Source: CAD feature listing. Evaluate the final solid. Frame: model axes, mm. Round coordinates to 2 decimals unless told otherwise and drop trailing zeros. Order: outer loops, then holes, each group sorted by start corner. A loop starts at its lowest first (then second) coordinate and runs counter-clockwise, first axis right, second up. Notation, with made-up numbers: (-34, 69.5) - (21, 69.5) arc R13 ccw to (21, 79.5) - close; hole circle Ø7 at (48, 33.5). An arc over 180 degrees is marked (long way). Use one line per item in the form item = value. Start each with the question number.
Q1. Pin query (flat end, axial travel): pin 1 Ø5 at (y, z) = (47, -16) entering from +X; pin 2 Ø5 at (y, z) = (79, 518.5) entering from +X; pin 3 Ø22.5 at (x, y) = (0, 0) entering from -Z; pin 4 Ø6 at (x, z) = (55, 151) entering from -Y. Return the tip coordinate at first contact, or that it passes through.
Q2. Cut plane A-A, the plane z = 119.5. Return the cut outline in (x, y), and give its area (3 significant figures).
Q3. Ray query, line 1 (Y direction, x = 0, z = 490); line 2 (X direction, y = -6.5, z = 469.5); line 3 (Y direction, x = 0, z = -408.75). Return the intervals inside material, ascending. Write a range as [from, to].
Q4. Draft query along Y for faces 1 (the cylindrical face through (-32.22, 245.394, 493.34)), 2 (the conical face through (-22.371, 100.745, -254.267)), 3 (the flat face through (-242, 57, 1000)). Return one class per face: released by +Y, released by -Y, zero draft, split by the parting line, or undercut.
Q5. Cut plane B-B, the plane z = -322. Return the cut outline in (x, y), and give its area (3 significant figures).
from build123d import *

# Parameters (mm, degrees)
F0_R     = 250
F1_DEPTH = 1000
F2_R     = 250
F4_T     = -2.5
F5_R     = 12.5
F6_DEPTH = 433.0137019922


# Not quite as in the source:
# - an extrude whose draft closes it to a point is written as a loft to that point


with BuildPart() as f1:
    # F0 (on Top) → F1 (new body)
    with BuildSketch(Plane.XY):
        Circle(F0_R)
    extrude(amount=F1_DEPTH)

    # F2 (on face) → F3 section 0
    with BuildSketch(Plane(origin=(0, 0, 0), x_dir=(1, 0, 0), z_dir=(0, 0, -1)), mode=Mode.PRIVATE) as f3_s0:
        Circle(F2_R)
    loft([f3_s0.sketch, Vertex(0, 0, -433.0127018922)], ruled=True)

    # F4
    f4_openings = [f1.faces().sort_by_distance(p)[0] for p in [
        (0, 0, 1000),
    ]]
    offset(amount=F4_T, openings=f4_openings)

    # F5 (on Top) → F6 (cut, through all)
    with BuildSketch(Plane.XY):
        Circle(F5_R)
    extrude(amount=-F6_DEPTH, mode=Mode.SUBTRACT)


solid = f1.part
Completed:
q1.pin_1 = 237.68
q1.pin_2 = 238.01
q1.pin_3 = through
q1.pin_4 = -244.53
q2.outline = circle Ø500 at (0, 0); hole circle Ø495 at (0, 0)
q2.area = 3,910 mm2
q3.line_1 = [-250, -247.5], [247.5, 250]
q3.line_2 = [-249.92, -247.41], [247.41, 249.92]
q3.line_3 = [-14.01, -12.5], [12.5, 14.01]
q4.face_1 = undercut
q4.face_2 = split by the parting line
q4.face_3 = zero draft
q5.outline = circle Ø128.19 at (0, 0); hole circle Ø122.41 at (0, 0)
q5.area = 1,140 mm2
